from build123d import *

# Parameters (mm, degrees)
SKETCH_1_W                   = 32.5
SKETCH_1_H                   = 36
EXTRUDE_1_DEPTH              = 18
SKETCH_2_W                   = 13
SKETCH_2_H                   = 26.5
CUT_EXTRUDE_1_DEPTH          = 42.282562905
HOLE_WIZARD_M2_3_AT_2_COUNT  = 2
HOLE_WIZARD_M2_3_AT_2_PITCH  = 21
CUT_EXTRUDE_3_DEPTH          = 40.555340979
CUT_EXTRUDE_3_DEPTH_BACK     = 40.555340979
SKETCH_4_R                   = 8.25
SKETCH_4_R_2                 = 1.2
SKETCH_18_R                  = 8
EXTRUDE_4_DEPTH              = 4
HOLE_WIZARD_M2_2_D           = 2.4
HOLE_WIZARD_M2_2_CBORE_D     = 4.2
HOLE_WIZARD_M2_2_CBORE_DEPTH = 1.45
SKETCH_19_R                  = 4.5
CUT_EXTRUDE_9_DEPTH          = 4
SKETCH_13_W                  = 37
SKETCH_13_H                  = 6
EXTRUDE_3_DEPTH              = 33
EXTRUDE_5_DEPTH              = 13
FILLET_1_R                   = 1
FILLET_2_R                   = 1
FILLET_3_R                   = 2
FILLET_4_R                   = 1
SKETCH_21_W                  = 27
SKETCH_21_H                  = 6
CUT_EXTRUDE_10_DEPTH         = 5


with BuildPart() as part:
    # ｽｹｯﾁ1 → ﾎﾞｽ - 押し出し1 (new body)
    with BuildSketch(Plane.XY):
        Rectangle(SKETCH_1_W, SKETCH_1_H)
    extrude(amount=EXTRUDE_1_DEPTH)

    # ｽｹｯﾁ2 → ｶｯﾄ - 押し出し1 (cut, through all)
    with BuildSketch(Plane(origin=(16.25, 0, 0), x_dir=(0, 0, -1), z_dir=(1, 0, 0))):
        with Locations((-6.5, 0)):
            Rectangle(SKETCH_2_W, SKETCH_2_H)
    extrude(amount=-CUT_EXTRUDE_1_DEPTH, mode=Mode.SUBTRACT)

    # ｽｹｯﾁ6 → M2 丸平ねじ用座ぐり穴3 (revolve, cut)
    with BuildSketch(Plane(origin=(13.75, 18, 6), x_dir=(0, 0, 1), z_dir=(1, 0, 0))):
        Polygon((0, 0), (0, 5.591204867), (1.4, 4.75), (1.4, 2), (2, 2), (2, 0), align=None)
    hole_wizard_m2_3 = revolve(axis=Axis((13.75, 24.35, 6), (0, -1, 0)), mode=Mode.SUBTRACT)

    # M2 丸平ねじ用座ぐり穴3 at 2: M2 丸平ねじ用座ぐり穴3 ×2
    with Locations(*[(-i * HOLE_WIZARD_M2_3_AT_2_PITCH, 0, 0) for i in range(1, HOLE_WIZARD_M2_3_AT_2_COUNT)]):
        add(hole_wizard_m2_3, mode=Mode.SUBTRACT)

    # ﾐﾗｰ1: M2 丸平ねじ用座ぐり穴3 across plane
    add(hole_wizard_m2_3.mirror(Plane.ZX), mode=Mode.SUBTRACT)

    # ﾐﾗｰ1 copy 1 sketch → ﾐﾗｰ1 copy 1 (revolve, cut)
    with BuildSketch(Plane(origin=(-7.25, -18, 6), x_dir=(0, 0, 1), z_dir=(1, 0, 0))):
        Polygon((0, 0), (0, -5.591204867), (1.4, -4.75), (1.4, -2), (2, -2), (2, 0), align=None)
    revolve(axis=Axis((-7.25, -24.35, 6), (0, -1, 0)), mode=Mode.SUBTRACT)

    # ｽｹｯﾁ4 → ｶｯﾄ - 押し出し3 (cut, two sides: drawn at the far end of the back side and taken through both)
    with BuildSketch(Plane.XZ.offset(-13.25).offset(-CUT_EXTRUDE_3_DEPTH_BACK)):
        with Locations((-7.25, -4.5)):
            Circle(SKETCH_4_R)
        with Locations((-7.25, 6)):
            Circle(SKETCH_4_R_2)
    extrude(amount=CUT_EXTRUDE_3_DEPTH + CUT_EXTRUDE_3_DEPTH_BACK, mode=Mode.SUBTRACT)

    # ｽｹｯﾁ18 → ﾎﾞｽ - 押し出し4 (add)
    with BuildSketch(Plane.XY.offset(18)):
        with Locations((-7.25, 0)):
            Circle(SKETCH_18_R)
    extrude(amount=EXTRUDE_4_DEPTH)

    # M2 丸平ねじ用座ぐり穴2 (through all)
    with Locations(Plane(origin=(0, 0, 13), x_dir=(-1, 0, 0), z_dir=(0, 0, -1))):
        with Locations((11.492640687, 4.242640687), (3.007359313, -4.242640687), (11.492640687, -4.242640687), (3.007359313, 4.242640687)):
            CounterBoreHole(HOLE_WIZARD_M2_2_D / 2, HOLE_WIZARD_M2_2_CBORE_D / 2, HOLE_WIZARD_M2_2_CBORE_DEPTH)

    # ｽｹｯﾁ19 → ｶｯﾄ - 押し出し9 (cut)
    with BuildSketch(Plane.XY.offset(22)):
        with Locations((-7.25, 0)):
            Circle(SKETCH_19_R)
    extrude(amount=-CUT_EXTRUDE_9_DEPTH, mode=Mode.SUBTRACT)

    # ｽｹｯﾁ13 → ﾎﾞｽ - 押し出し3 (add)
    with BuildSketch(Plane(origin=(0, 18, 0), x_dir=(1, 0, 0), z_dir=(0, 1, 0))):
        with Locations((-7.25, -15)):
            Rectangle(SKETCH_13_W, SKETCH_13_H)
    extrude(amount=EXTRUDE_3_DEPTH)

    # ｽｹｯﾁ20 → ﾎﾞｽ - 押し出し5 (add)
    with BuildSketch(Plane(origin=(0, 51, 0), x_dir=(1, 0, 0), z_dir=(0, 1, 0))):
        with BuildLine():
            Line((11.25, -12), (11.25, -99))
            ThreePointArc((11.25, -99), (8.613961031, -105.363961031), (2.25, -108))
            Line((2.25, -108), (-16.75, -108))
            ThreePointArc((-16.75, -108), (-23.113961031, -105.363961031), (-25.75, -99))
            Line((-25.75, -99), (-25.75, -12))
            Line((-25.75, -12), (-20.75, -12))
            Line((-20.75, -12), (-20.75, -99))
            ThreePointArc((-20.75, -99), (-19.578427125, -101.828427125), (-16.75, -103))
            Line((-16.75, -103), (2.25, -103))
            ThreePointArc((2.25, -103), (5.078427125, -101.828427125), (6.25, -99))
            Line((6.25, -99), (6.25, -12))
            Line((6.25, -12), (11.25, -12))
        make_face()
    extrude(amount=EXTRUDE_5_DEPTH)

    # ﾌｨﾚｯﾄ1
    fillet_1_edges = [part.edges().sort_by_distance(p)[0] for p in [
        (-23.25, 51, 18),
        (8.75, 51, 18),
    ]]
    fillet(fillet_1_edges, radius=FILLET_1_R)

    # ﾌｨﾚｯﾄ2
    fillet_2_edges = [part.edges().sort_by_distance(p)[0] for p in [
        (8.75, 64, 12),
        (-23.25, 64, 12),
    ]]
    fillet(fillet_2_edges, radius=FILLET_2_R)

    # ﾌｨﾚｯﾄ3
    fillet_3_edges = [part.edges().sort_by_distance(p)[0] for p in [
        (-16.25, 18, 15),
    ]]
    fillet(fillet_3_edges, radius=FILLET_3_R)

    # ﾌｨﾚｯﾄ4
    fillet_4_edges = [part.edges().sort_by_distance(p)[0] for p in [
        (-11.75, 0, 18),
        (-15.25, 0, 18),
    ]]
    fillet(fillet_4_edges, radius=FILLET_4_R - 0.0001)  # a hair under: the kernel refuses the full size

    # ｽｹｯﾁ21 → ｶｯﾄ - 押し出し10 (cut)
    with BuildSketch(Plane(origin=(0, 51, 0), x_dir=(1, 0, 0), z_dir=(0, 1, 0))):
        with Locations((-7.25, -15)):
            Rectangle(SKETCH_21_W, SKETCH_21_H)
    extrude(amount=-CUT_EXTRUDE_10_DEPTH, mode=Mode.SUBTRACT)


solid = part.part
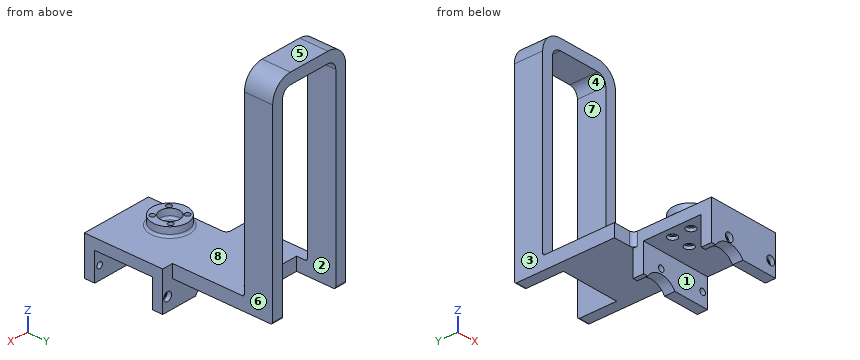
Source: CAD feature listing. Evaluate the final solid. Frame: model axes, mm. Face numbers are marked on the shaded views. A direction names the side the tool comes from. Round coordinates to 2 decimals unless told otherwise and drop trailing zeros. Loops run counter-clockwise (first coordinate to the right, second up) from the corner with the lowest first, then second, coordinate; pieces in that order, holes last. Notation, with made-up numbers: M -29,87.25 L -12,87.25 A22 cw -12,101.25 Z; hole C 88,84 d9. An arc over 180 degrees is marked long. Return JSON: item names as keys, results as strings. Group by question number.
1. Mould query, pull axis X, two halves, no side actions, for the marked faces 6, 7 and 8. Classes: released by +X, released by -X, zero draft, split by the parting line, or undercut.
2. Pin query (flat end, axial travel): pin 1 (2 mm diameter, centred on x = -6.5, z = 5, fed in from +Y); pin 2 (5 mm diameter, centred on x = 2.5, y = 36, fed in from +Z); pin 3 (3 mm diameter, centred on x = -3.01, y = 4.24, fed in from +Z). Return the tip coordinate at first contact, or that it passes through.
3. Material intervals for line 1 along X through (y, z) = (16.45, 6); line 2 along Z through (x, y) = (-7.25, -17.1); line 3 along Z through (x, y) = (-21.5, 41.5), sorted ascending. Write a range as from..to.
4. Section query A-A on z = 80. Output: boundary loops of the cut face in (x, y).
5. Section query D-D on x = -23. Output: boundary loops of the cut face in (y, z), and give its area (3 significant figures).
6. Reachability of the marked faces 1, 2, 3, 4 and 5 from +Z, -Z, +X, -X, +Y, -Y: full face, straight path, thin tool, end or side. Return the list, or none.
7. Section query B-B on x = 13.75. Output: boundary loops of the cut face in (y, z), and give its area (3 significant figures).
8. Section query C-C on y = 59.5. Output: boundary loops of the cut face in (x, z).
Checks:
{
 "1": {"face 6": "released by +X", "face 7": "undercut", "face 8": "zero draft"},
 "2": {"pin 1": "stops at y = 18", "pin 2": "stops at z = 18", "pin 3": "stops at z = 22"},
 "3": {"line 1": "x = -16.25..-9.25, -5.25..11.75, 15.75..16.25", "line 2": "z = 3.75..4, 8..18", "line 3": "z = 12..18"},
 "4": {"outline": "M -25.75,51 L -20.75,51 L -20.75,64 L -25.75,64 Z; M 6.25,51 L 11.25,51 L 11.25,64 L 6.25,64 Z"},
 "5": {"outline": "M 18,12 L 63,12 A1 ccw 64,13 L 64,105.48 L 51,105.48 L 51,19 A1 cw 50,18 L 18,18 Z", "area": "1,410 mm²"},
 "6": {"face 1": "-Z, +X, -X", "face 2": "-Z, +Y", "face 3": "+Z, -Z, -X, +Y, -Y", "face 4": "-Z, +Y, -Y", "face 5": "+Z, +X, -X, +Y, -Y"},
 "7": {"outline": "M -18,0 L -13.25,0 L -13.25,4.6 L -16,4.6 L -16,4 L -18,4 Z; M -18,8 L -16,8 L -16,7.4 L -13.25,7.4 L -13.25,13 L 13.25,13 L 13.25,7.4 L 16,7.4 L 16,8 L 18,8 L 18,18 L -18,18 Z; M 13.25,0 L 18,0 L 18,4 L 16,4 L 16,4.6 L 13.25,4.6 Z", "area": "272 mm²"},
 "8": {"outline": "M -25.75,12 L -20.75,12 L -20.75,99 A4 cw -16.75,103 L 2.25,103 A4 cw 6.25,99 L 6.25,12 L 11.25,12 L 11.25,99 A9 ccw 2.25,108 L -16.75,108 A9 ccw -25.75,99 Z"}
}
